The model under review builds one solid part; all positions refer to its coordinate system, in mm. A direction names the side the tool comes from. Give positions to 0.01 mm unless a question says otherwise; leave off trailing zeros. Loops run counter-clockwise (first coordinate to the right, second up) from the corner with the lowest first, then second, coordinate; pieces in that order, holes last. Notation, with made-up numbers: M 79.25,-16 L 96.25,-16 A21 ccw 96.25,15 Z; hole C 75.5,22 d4. An arc over 180 degrees is marked long. One line per item, written item: value. Start each with the question number.
Q1. We need section D-D on y = 1.9. Write out the cut boundary in (x, z), plus the area to 3 significant figures.
Q2. To check wall thickness, follow line 1 along X through (y, z) = (3.4, 8.5); line 2 along X through (y, z) = (2.2, 6); line 3 along Y through (x, z) = (-0.2, 6.5). State the ranges of each line that lie inside material, in increasing order. Write a range as from..to.
Q3. We need section C-C on z = 2.25. Write out the cut boundary in (x, y).
Q4. For pin 1 (2 mm diameter, centred on y = 2.5, z = 5, fed in from +X); pin 2 (1.3 mm diameter, centred on x = 0, z = 10.5, fed in from -Y); pin 3 (1.1 mm diameter, centred on y = 3.5, z = 4.5, fed in from -X), all flat-tipped, find the tip position at first contact; note any pin that passes through.
Q5. We need section B-B on y = 3.4. Write out the cut boundary in (x, z).
Q6. For faces 4 (the face through (0, 1, 10)), 5 (the face through (2.5, 1, 4)), 6 (the face through (-1.9, 0.9, 3.3)), 7 (the face through (0, 3, 6)), 8 (the face through (2, 0.9, 3.3)), list the 3-axis set-ups (+Z, -Z, +X, -X, +Y, -Y) from which the entire face can be reached by the end or side of a thin tool; tool diameter is ignored.
Q7. We need section A-A on x = 0.1. Write out the cut boundary in (y, z), plus the area to 3 significant figures.
Q8. Mouldability with a two-part tool opening along X and no side actions: class faces 1 (the face through (-0.75, 3.5, 5.4)), 2 (the face through (-0.02, 0.575, 2.353)), 3 (the face through (1.4, 2, 7)) as released by +X, released by -X, zero draft, split by the parting line, or undercut.
```python
from build123d import *

# Parameters (mm, degrees)
PROFILE_DEPTH         = 1.4
PIVOTTABS_R           = 0.7
PIVOTTAB_DEPTH        = 2.5
TOPCUTS_W             = 1.5
TOPCUTS_H             = 15
TOPCUT_DEPTH          = 1
PIVOTSLANT_DEPTH      = 16.724185194
PIVOTSLANT_DEPTH_BACK = 16.724185194
PIVOTSLANTF_R         = 0.2
BOTTOMCAVITYS_W       = 1.6
BOTTOMCAVITYS_H       = 8.2736695
BOTTOMCAVITY_DEPTH    = 1
BOTTOMCAVITYF_R       = 0.2


with BuildPart() as part:
    # ProfileS → Profile (new, symmetric)
    with BuildSketch(Plane(origin=(0, 0, 0), x_dir=(0, 0, -1), z_dir=(1, 0, 0))):
        with BuildLine():
            Line((0, 0), (-15, 0))
            Line((-15, 0), (-15, 0.608001659))
            ThreePointArc((-15, 0.608001659), (-14.968678289, 0.715461581), (-14.884523652, 0.789263217))
            Line((-14.884523652, 0.789263217), (-8.2, 3.906307787))
            ThreePointArc((-8.2, 3.906307787), (-7.993821352, 3.976296007), (-7.777381738, 4))
            Line((-7.777381738, 4), (-3, 4))
            ThreePointArc((-3, 4), (-0.878679656, 3.121320344), (0, 1))
            Line((0, 1), (0, 0))
        make_face()
    extrude(amount=PROFILE_DEPTH, both=True)

    # PivotTabS → PivotTab (add, symmetric)
    with BuildSketch(Plane(origin=(0, 0, 0), x_dir=(0, 0, -1), z_dir=(1, 0, 0))):
        with Locations(Location((-4, 0.9, 0), (0, 0, 180))):
            Circle(PIVOTTABS_R)
    extrude(amount=PIVOTTAB_DEPTH, both=True)

    # TopCutS → TopCut (cut)
    with BuildSketch(Plane(origin=(0, 4, 18.512140764), x_dir=(1, 0, 0), z_dir=(0, -1, 0))):
        with Locations((0, -11.012140764)):
            Rectangle(TOPCUTS_W, TOPCUTS_H)
    extrude(amount=TOPCUT_DEPTH, mode=Mode.SUBTRACT)

    # PivotSlantS → PivotSlant (cut, two sides: drawn at the far end of the back side and taken through both)
    with BuildSketch(Plane(origin=(0, 0, 0), x_dir=(0, 0, -1), z_dir=(1, 0, 0)).offset(-PIVOTSLANT_DEPTH_BACK)):
        Polygon((-4.5, 0), (0, 1.205771366), (0, 0), align=None)
    extrude(amount=PIVOTSLANT_DEPTH + PIVOTSLANT_DEPTH_BACK, mode=Mode.SUBTRACT)

    # PivotSlantF
    pivotslantf_edges = [part.edges().sort_by_distance(p)[0] for p in [
        (0, 0, 15),
        (0, 0, 4.5),
        (0, 1.203912318, 0.006938062),
    ]]
    fillet(pivotslantf_edges, radius=PIVOTSLANTF_R)

    # BottomCavityS → BottomCavity (cut)
    with BuildSketch(Plane(origin=(0, 0, 0), x_dir=(-1, 0, 0), z_dir=(0, -1, 0))):
        with Locations((0, -9.66316525)):
            Rectangle(BOTTOMCAVITYS_W, BOTTOMCAVITYS_H)
    extrude(amount=-BOTTOMCAVITY_DEPTH, mode=Mode.SUBTRACT)

    # BottomCavityF
    bottomcavityf_edges = [part.edges().sort_by_distance(p)[0] for p in [
        (-0.8, 1, 9.66316525),
        (-0.8, 0.5, 5.5263305),
        (0, 1, 13.8),
        (-0.8, 0.5, 13.8),
        (0.8, 1, 9.66316525),
        (0.8, 0.5, 13.8),
        (0, 1, 5.5263305),
        (0.8, 0.5, 5.5263305),
    ]]
    fillet(bottomcavityf_edges, radius=BOTTOMCAVITYF_R)


solid = part.part
```
Solved:
1. outline: M -1.4,0.14 L 1.4,0.14 L 1.4,12.5 L -1.4,12.5 Z
1. area: 34.6 mm2
2. line 1: -1.4..-0.75, 0.75..1.4
2. line 2: -1.4..1.4
2. line 3: 1..3
3. outline: M -1.4,0.6 L 1.4,0.6 L 1.4,3.9 L 0.75,3.9 L 0.75,3 L -0.75,3 L -0.75,3.9 L -1.4,3.9 Z
4. pin 1: x = 1.4
4. pin 2: y = 0.99
4. pin 3: x = -1.4
5. outline: M -1.4,1.2 L -0.75,1.2 L -0.75,9.29 L -1.4,9.29 Z; M 0.75,1.2 L 1.4,1.2 L 1.4,9.29 L 0.75,9.29 Z
6. face 4: -Y
6. face 5: +Z, -Z, +X, +Y, -Y
6. face 6: -X
6. face 7: +Z, -Z, +Y
6. face 8: +X
7. outline: M 0,4.53 A0.2 ccw 0.01,4.47 L 1.16,0.17 A0.2 ccw 1.38,0.02 A3 ccw 3,0.76 L 3,10.14 L 0.79,14.88 A0.2 ccw 0.61,15 L 0.2,15 A0.2 ccw 0,14.8 L 0,13.8 L 0.8,13.8 A0.2 cw 1,13.6 L 1,5.73 A0.2 cw 0.8,5.53 L 0,5.53 Z
7. area: 28.0 mm2
8. face 1: undercut
8. face 2: zero draft
8. face 3: released by +X
